Can you work these out from the model? Positions are in its coordinate system, mm. A direction names the side the tool comes from. Give positions to 0.01 mm unless a question says otherwise; leave off trailing zeros. Loops run counter-clockwise (first coordinate to the right, second up) from the corner with the lowest first, then second, coordinate; pieces in that order, holes last. Notation, with made-up numbers: (4.5, 71.25) - (55.5, 71.25) arc R18 ccw to (55.5, 77.25) - close; hole circle Ø9 at (5.25, -14.5). An arc over 180 degrees is marked (long way). Answer as a JSON object with one key per item and string values.
```python
from build123d import *

# Parameters (mm, degrees)
BOSS_EXTRUDE1_START = 17.075
SKETCH1_W           = 16.2
SKETCH1_H           = 32.8
BOSS_EXTRUDE1_DEPTH = 10.275
BOSS_EXTRUDE2_START = -12.425
SKETCH2_W           = 16.2
SKETCH2_H           = 32.8
BOSS_EXTRUDE2_DEPTH = 10.275
BOSS_EXTRUDE3_START = 7.3
SKETCH3_W           = 16.2
SKETCH3_H           = 20.55
BOSS_EXTRUDE3_DEPTH = 0.5
CUT_EXTRUDE1_START  = 18.725
SKETCH4_W           = 13
SKETCH4_H           = 23.2
CUT_EXTRUDE1_DEPTH  = 8.625
CUT_EXTRUDE2_START  = 24.35
SKETCH5_R           = 1
CUT_EXTRUDE2_DEPTH  = 3
CUT_EXTRUDE3_START  = 24.35
SKETCH6_R           = 1
CUT_EXTRUDE3_DEPTH  = 3
CUT_EXTRUDE4_START  = 8.1
SKETCH7_R           = 3.15
CUT_EXTRUDE4_DEPTH  = 1.3
CUT_EXTRUDE5_START  = 8.5
SKETCH8_W           = 4.4
SKETCH8_H           = 6
CUT_EXTRUDE5_DEPTH  = 2.4
CUT_EXTRUDE6_START  = -10.775
SKETCH9_W           = 13
SKETCH9_H           = 23.2
CUT_EXTRUDE6_DEPTH  = 8.625
CUT_EXTRUDE7_START  = -5.15
SKETCH10_R          = 1
CUT_EXTRUDE7_DEPTH  = 3
CUT_EXTRUDE8_START  = -5.15
SKETCH11_R          = 1
CUT_EXTRUDE8_DEPTH  = 3
CUT_EXTRUDE9_START  = -21.4
SKETCH12_R          = 3.15
CUT_EXTRUDE9_DEPTH  = 1.3
CUT_EXTRUDE10_START = 10
SKETCH13_W          = 4.4
SKETCH13_H          = 6
CUT_EXTRUDE10_DEPTH = 2.4


with BuildPart() as part:
    # Sketch1 → Boss-Extrude1 (new, symmetric)
    with BuildSketch(Plane(origin=(0, 0, 0), x_dir=(1, 0, 0), z_dir=(0, 1, 0)).offset(BOSS_EXTRUDE1_START)):
        with Locations((0, 5.5)):
            Rectangle(SKETCH1_W, SKETCH1_H)
    extrude(amount=BOSS_EXTRUDE1_DEPTH, both=True)

    # Sketch2 → Boss-Extrude2 (add, symmetric)
    with BuildSketch(Plane.XY.offset(BOSS_EXTRUDE2_START)):
        with Locations((-16.2, 24)):
            Rectangle(SKETCH2_W, SKETCH2_H)
    extrude(amount=BOSS_EXTRUDE2_DEPTH, both=True)

    # Sketch3 → Boss-Extrude3 (add, symmetric)
    with BuildSketch(Plane(origin=(0, 0, 0), x_dir=(1, 0, 0), z_dir=(0, 1, 0)).offset(BOSS_EXTRUDE3_START)):
        with Locations((-16.2, 12.425)):
            Rectangle(SKETCH3_W, SKETCH3_H)
    extrude(amount=BOSS_EXTRUDE3_DEPTH, both=True)

    # Sketch4 → Cut-Extrude1 (cut, symmetric)
    with BuildSketch(Plane(origin=(0, 0, 0), x_dir=(1, 0, 0), z_dir=(0, 1, 0)).offset(CUT_EXTRUDE1_START)):
        with Locations((0, 5.5)):
            Rectangle(SKETCH4_W, SKETCH4_H)
    extrude(amount=CUT_EXTRUDE1_DEPTH, both=True, mode=Mode.SUBTRACT)

    # Sketch5 → Cut-Extrude2 (cut, symmetric)
    with BuildSketch(Plane(origin=(0, 0, 0), x_dir=(1, 0, 0), z_dir=(0, 1, 0)).offset(CUT_EXTRUDE2_START)):
        with Locations(Location((0, 19.25, 0), (0, 0, 270))):
            Circle(SKETCH5_R)
    extrude(amount=CUT_EXTRUDE2_DEPTH, both=True, mode=Mode.SUBTRACT)

    # Sketch6 → Cut-Extrude3 (cut, symmetric)
    with BuildSketch(Plane(origin=(0, 0, 0), x_dir=(1, 0, 0), z_dir=(0, 1, 0)).offset(CUT_EXTRUDE3_START)):
        with Locations(Location((0, -8.25, 0), (0, 0, 270))):
            Circle(SKETCH6_R)
    extrude(amount=CUT_EXTRUDE3_DEPTH, both=True, mode=Mode.SUBTRACT)

    # Sketch7 → Cut-Extrude4 (cut, symmetric)
    with BuildSketch(Plane(origin=(0, 0, 0), x_dir=(1, 0, 0), z_dir=(0, 1, 0)).offset(CUT_EXTRUDE4_START)):
        with Locations(Location((0, 0, 0), (0, 0, 270))):
            Circle(SKETCH7_R)
    extrude(amount=CUT_EXTRUDE4_DEPTH, both=True, mode=Mode.SUBTRACT)

    # Sketch8 → Cut-Extrude5 (cut, symmetric)
    with BuildSketch(Plane.XY.offset(CUT_EXTRUDE5_START)):
        with Locations((0, 13.1)):
            Rectangle(SKETCH8_W, SKETCH8_H)
    extrude(amount=CUT_EXTRUDE5_DEPTH, both=True, mode=Mode.SUBTRACT)

    # Sketch9 → Cut-Extrude6 (cut, symmetric)
    with BuildSketch(Plane.XY.offset(CUT_EXTRUDE6_START)):
        with Locations((-16.2, 24)):
            Rectangle(SKETCH9_W, SKETCH9_H)
    extrude(amount=CUT_EXTRUDE6_DEPTH, both=True, mode=Mode.SUBTRACT)

    # Sketch10 → Cut-Extrude7 (cut, symmetric)
    with BuildSketch(Plane.XY.offset(CUT_EXTRUDE7_START)):
        with Locations((-16.2, 37.75)):
            Circle(SKETCH10_R)
    extrude(amount=CUT_EXTRUDE7_DEPTH, both=True, mode=Mode.SUBTRACT)

    # Sketch11 → Cut-Extrude8 (cut, symmetric)
    with BuildSketch(Plane.XY.offset(CUT_EXTRUDE8_START)):
        with Locations((-16.2, 10.25)):
            Circle(SKETCH11_R)
    extrude(amount=CUT_EXTRUDE8_DEPTH, both=True, mode=Mode.SUBTRACT)

    # Sketch12 → Cut-Extrude9 (cut, symmetric)
    with BuildSketch(Plane.XY.offset(CUT_EXTRUDE9_START)):
        with Locations((-16.2, 18.5)):
            Circle(SKETCH12_R)
    extrude(amount=CUT_EXTRUDE9_DEPTH, both=True, mode=Mode.SUBTRACT)

    # Sketch13 → Cut-Extrude10 (cut, symmetric)
    with BuildSketch(Plane(origin=(0, 0, 0), x_dir=(1, 0, 0), z_dir=(0, 1, 0)).offset(CUT_EXTRUDE10_START)):
        with Locations((-16.2, 16.4)):
            Rectangle(SKETCH13_W, SKETCH13_H)
    extrude(amount=CUT_EXTRUDE10_DEPTH, both=True, mode=Mode.SUBTRACT)


solid = part.part
```
1) Imagine slicing it at D-D on y = 18.5. Write out the boundary of the cut face in (x, z), and give its area (3 significant figures).
Check sheet entries:
{"outline": "(-24.3, -22.7) - (-19.35, -22.7) - (-19.35, -20.1) - (-13.05, -20.1) - (-13.05, -22.7) - (-8.1, -22.7) - (-8.1, -21.9) - (8.1, -21.9) - (8.1, 10.9) - (-8.1, 10.9) - (-8.1, -2.15) - (-9.7, -2.15) - (-9.7, -19.4) - (-22.7, -19.4) - (-22.7, -2.15) - (-24.3, -2.15) - close; hole (-6.5, -17.1) - (6.5, -17.1) - (6.5, 6.1) - (-6.5, 6.1) - close", "area": "322 mm2"}
2) Imagine slicing it at A-A on x = 0. Write out the boundary of the cut face in (y, z).
Check sheet entries:
{"outline": "(6.8, -21.9) - (27.35, -21.9) - (27.35, -20.25) - (21.35, -20.25) - (21.35, -18.25) - (27.35, -18.25) - (27.35, -17.1) - (10.1, -17.1) - (10.1, 10.9) - (6.8, 10.9) - (6.8, 3.15) - (9.4, 3.15) - (9.4, -3.15) - (6.8, -3.15) - close; (16.1, 6.1) - (27.35, 6.1) - (27.35, 7.25) - (21.35, 7.25) - (21.35, 9.25) - (27.35, 9.25) - (27.35, 10.9) - (16.1, 10.9) - close"}
3) Which directions (+Z, -Z, +X, -X, +Y, -Y) give clear straight access to the entire face, cutting with the end or side of a thin tool? Please do faces 4 (the flat face through (-2.2, 13, 9)), 5 (the flat face through (0, 9.4, 0)), 6 (the flat face through (6.5, 19, -5)), 7 (the flat face through (-16, 7.6, -16)), 8 (the flat face through (-7, 27.35, -6)).
Check sheet entries:
{"face 4": "+Z", "face 5": "-Y", "face 6": "+Y", "face 7": "none", "face 8": "+Z, -Z, +X, +Y"}
4) If we mould it in two halves opening along X, with no side actions, what happens to faces 1 (the flat face through (-8, 6.8, -10)), 2 (the flat face through (0, 21.35, 8)), 3 (the flat face through (-8.1, 17, 4))? For each: released by +X, released by -X, zero draft, split by the parting line, or undercut.
Check sheet entries:
{"face 1": "zero draft", "face 2": "undercut", "face 3": "released by -X"}
5) Imagine slicing it at B-B on z = 8.25. Write out the boundary of the cut face in (x, y), and give its area (3 significant figures).
Check sheet entries:
{"outline": "(-8.1, 6.8) - (8.1, 6.8) - (8.1, 27.35) - (1, 27.35) - (1, 21.35) - (-1, 21.35) - (-1, 27.35) - (-8.1, 27.35) - close; hole (-2.2, 10.1) - (2.2, 10.1) - (2.2, 16.1) - (-2.2, 16.1) - close", "area": "295 mm2"}
6) I need wall thicknesses on L1, parallel to Y at x = -18, z = -7; L2, parallel to Z at x = 2, y = 25; L3, parallel to Z at x = -0.5, y = 23. Which ranges of each line are inside material? Lowest first, please.
Check sheet entries:
{"L1": "6.8 to 12.4, 35.6 to 40.4", "L2": "-21.9 to -17.1, 6.1 to 10.9", "L3": "-21.9 to -20.12, -18.38 to -17.1, 6.1 to 7.38, 9.12 to 10.9"}
7) I'm going to push flat-ended pins straight in: P1, Ø12, axis at x = 2, z = -5.5, coming from the +Y side; P2, Ø8, axis at x = -1.5, y = 19.5, coming from the -Z side; P3, Ø10.5, axis at y = 14.5, z = 7, coming from the -X side; P4, Ø12, axis at x = -18.5, z = 5.5, coming from the -Y side. Where does each tip first touch, or does it pass through?
Check sheet entries:
{"P1": "y = 27.35", "P2": "z = -21.9", "P3": "x = -8.1", "P4": "through"}
8) Imagine slicing it at C-C on y = 32. Write out the boundary of the cut face in (x, z), and give its area (3 significant figures).
Check sheet entries:
{"outline": "(-24.3, -22.7) - (-8.1, -22.7) - (-8.1, -2.15) - (-9.7, -2.15) - (-9.7, -19.4) - (-22.7, -19.4) - (-22.7, -2.15) - (-24.3, -2.15) - close", "area": "109 mm2"}
